The model under review builds one solid part; all positions refer to its coordinate system, in mm. Face numbers are marked on the shaded views. A direction names the side the tool comes from. Coordinates: 2 decimals unless noted, no trailing zeros. Loops run counter-clockwise (first coordinate to the right, second up) from the corner with the lowest first, then second, coordinate; pieces in that order, holes last. Notation, with made-up numbers: (43, 12.25) -> (71, 12.25) arc R21 cw to (71, 28.25) -> close; hole circle Ø11 at (39.25, 63). An arc over 180 degrees is marked (long way). One line per question, with ' | ' between items. Start each with the question number.
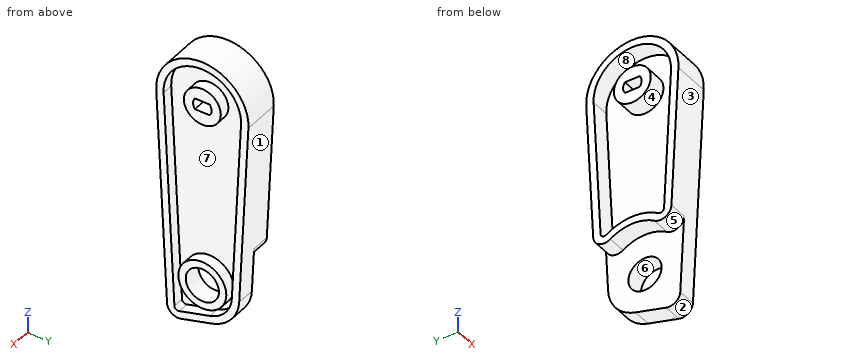
from build123d import *

# Parameters (mm, degrees)
F1_DEPTH  = 10
F3_DEPTH  = 5
F4_R      = 4.5
F5_DEPTH  = 10.001
F6_T      = -2
F7_R      = 1
F8_R      = 3
F10_DEPTH = 2
F11_R     = 5
F12_DEPTH = 10
F14_DEPTH = 10.001


with BuildPart() as f1:
    # F0 (on Right) → F1 (new body)
    with BuildSketch(Plane.YZ):
        with BuildLine():
            Line((9.9874921777, -50.5), (12.4843652221, -0.625))
            ThreePointArc((12.4843652221, -0.625), (0, 12.5), (-12.4843652221, -0.625))
            Line((-12.4843652221, -0.625), (-9.3685649734, -62.863061223))
            Line((-9.3685649734, -62.863061223), (2.588190451, -59.6592582629))
            ThreePointArc((2.588190451, -59.6592582629), (7.7788142654, -56.2841108061), (9.9874921777, -50.5))
        make_face()
    extrude(amount=F1_DEPTH)

    # F2 (on Right) → F3 (cut)
    with BuildSketch(Plane.YZ):
        with BuildLine():
            ThreePointArc((11, -50), (0, -39), (-11, -50))
            Line((-11, -50), (-11, -80))
            Line((-11, -80), (11, -80))
            Line((11, -80), (11, -50))
        make_face()
    extrude(amount=F3_DEPTH, mode=Mode.SUBTRACT)

    # F4 (on Right) → F5 (cut, through all)
    with BuildSketch(Plane.YZ):
        with Locations((0, -50)):
            Circle(F4_R)
    extrude(amount=F5_DEPTH, mode=Mode.SUBTRACT)

    # F6
    f6_openings = [f1.faces().sort_by_distance(p)[0] for p in [
        (0, 0, -14.700163),
        (10, -0.155944, -22.13999),
    ]]
    offset(amount=F6_T, openings=f6_openings, kind=Kind.INTERSECTION)

    # F7
    f7_edges = [f1.edges().sort_by_distance(p)[0] for p in [
        (3.5, 8.502341, -40.165866),
        (3.5, -8.502341, -40.165866),
        (8.5, -7.494852, -60.290449),
    ]]
    fillet(f7_edges, radius=F7_R)

    # F8
    f8_edges = [f1.edges().sort_by_distance(p)[0] for p in [
        (2.5, 10.216621, -45.923156),
        (2.5, -10.216621, -45.923156),
        (7.5, -9.368565, -62.863061),
    ]]
    fillet(f8_edges, radius=F8_R)

    # F9 (on face) → F10 (join)
    with BuildSketch(Plane(origin=(5, 0, 0), x_dir=(0, -1, 0), z_dir=(-1, 0, 0))):
        with BuildLine():
            Line((-10.4868667866, -0.525), (-8.5962115248, -38.2908092756))
            ThreePointArc((-8.5962115248, -38.2908092756), (-8.0535356457, -39.1307514702), (-7.054786428, -39.0807514702))
            ThreePointArc((-7.054786428, -39.0807514702), (0, -37), (7.054786428, -39.0807514702))
            ThreePointArc((7.054786428, -39.0807514702), (8.0535356457, -39.1307514702), (8.5962115248, -38.2908092756))
            Line((8.5962115248, -38.2908092756), (10.4868667866, -0.525))
            ThreePointArc((10.4868667866, -0.525), (0, 10.5), (-10.4868667866, -0.525))
        make_face()
    extrude(amount=-F10_DEPTH)

    # F11 (on Right) → F12 (join)
    with BuildSketch(Plane.YZ):
        Circle(F11_R)
    extrude(amount=F12_DEPTH)

    # F13 (on Right) → F14 (cut, through all)
    with BuildSketch(Plane.YZ):
        with BuildLine():
            Line((-2, -1.5), (2, -1.5))
            ThreePointArc((2, -1.5), (2.5, 0), (2, 1.5))
            Line((2, 1.5), (-2, 1.5))
            ThreePointArc((-2, 1.5), (-2.5, 0), (-2, -1.5))
        make_face()
    extrude(amount=F14_DEPTH, mode=Mode.SUBTRACT)


solid = f1.part
1) Insertion check: pin 1 Ø4.5 at (x, y) = (4, -0.5) entering from -Z; pin 2 Ø1 at (x, z) = (6, -24) entering from -Y; pin 3 Ø4 at (x, y) = (8.5, -8) entering from +Z. Each pin has a flat end and moves straight along its axis. Give the tip position at first contact, or say it passes through.
2) Consider section B-B, the plane y = 0. Give the number of separate pieces and of enclosed holes in the cut face, plus the area to 3 significant figures.
3) Consider section A-A, the plane x = 6.25. Write out the cut boundary in (y, z) (1 decimal), plus the area to 3 significant figures.
4) Wall thickness on L1, parallel to Z at x = 2.25, y = 3; L2, parallel to Z at x = 6.6, y = 0; L3, parallel to Y at x = 7.2, z = -50: over which ranges is each line inside the solid? List them lowest first.
5) Consider section C-C, the plane z = -22. Write out the cut boundary in (x, y).
6) Mouldability with a two-part tool opening along Y and no side actions: class the marked faces 1, 2, 3 and 4 as +Y half, -Y half, draft (parallel to the pull), parting line (faces both ways), or undercut.
7) Consider section D-D, the plane z = -13. Write out the cut boundary in (x, y).
8) Machinability: for the marked faces 5, 6, 7 and 8, which of the approach directions +Z, -Z, +X, -X, +Y, -Y give a long, thin tool a straight path to every point of the face, cutting with its end or side? Answer none if there is none.
Filled sheet:
1) pin 1: z = -61.03 | pin 2: y = -11.34 | pin 3: z = 10.97
2) separate pieces: 3 | enclosed holes: 0 | area: 222 mm^2
3) outline: (-12.5, -0.6) -> (-9.6, -59.2) arc R3 ccw to (-5.8, -61.9) -> (2.6, -59.7) arc R10 ccw to (10, -50.5) -> (12.5, -0.6) arc R12.5 ccw (long way) to start; hole circle Ø9 at (0, -50); hole (-2, -1.5) -> (2, -1.5) arc R2.5 ccw to (2, 1.5) -> (-2, 1.5) arc R2.5 ccw to start | area: 1,480 mm^2
4) L1: -39.42 to -37.35, -4 to 4, 10.06 to 12.13 | L2: -60.35 to -54.5, -45.5 to -1.5, 1.5 to 12.5 | L3: -10.01 to -8.01, -6.5 to -4.5, 4.5 to 6.5, 8.01 to 10.01
5) outline: (0, -11.41) -> (10, -11.41) -> (10, -9.41) -> (7, -9.41) -> (7, 9.41) -> (10, 9.41) -> (10, 11.41) -> (0, 11.41) -> (0, 9.41) -> (5, 9.41) -> (5, -9.41) -> (0, -9.41) -> close
6) face 1: +Y half | face 2: parting line | face 3: -Y half | face 4: undercut
7) outline: (0, -11.86) -> (10, -11.86) -> (10, -9.86) -> (7, -9.86) -> (7, 9.86) -> (10, 9.86) -> (10, 11.86) -> (0, 11.86) -> (0, 9.86) -> (5, 9.86) -> (5, -9.86) -> (0, -9.86) -> close
8) face 5: -Z, -X | face 6: +X, -X | face 7: +X | face 8: -X
